```python
from build123d import *

# Parameters (mm, degrees)
SKETCH_1_W           = 50
SKETCH_1_H           = 50
EXTRUDE_1_DEPTH      = 50
SKETCH_6_R           = 12
SKETCH_6_R_2         = 11
EXTRUDE_3_DEPTH      = 9
CUT_EXTRUDE_5_REACH  = 83.277
CUT_EXTRUDE_6_REACH  = 83.277
SKETCH_20_W          = 48
SKETCH_20_H          = 48
CUT_EXTRUDE_7_DEPTH  = 30
CUT_EXTRUDE_START    = -29
SKETCH_21_R          = 11
CUT_EXTRUDE_9_DEPTH  = 29
SKETCH_28_W          = 48
SKETCH_28_H          = 48
CUT_EXTRUDE_11_DEPTH = 18
CUT_EXTRUDE_11_DRAFT = -33


with BuildPart() as part:
    # Эскиз1 → Бобышка-Вытянуть1 (new body)
    with BuildSketch(Plane.XY):
        Rectangle(SKETCH_1_W, SKETCH_1_H)
    extrude(amount=EXTRUDE_1_DEPTH)

    # Эскиз6 → Бобышка-Вытянуть3 (add)
    with BuildSketch(Plane.XY.offset(50)):
        Circle(SKETCH_6_R)
        Circle(SKETCH_6_R_2, mode=Mode.SUBTRACT)
    extrude(amount=EXTRUDE_3_DEPTH)

    # Вырез-Вытянуть5: up to this face of the body (flat: up to its plane)
    cut_extrude_5_end = Plane(part.part.faces().sort_by_distance((0, 25, 25))[0])
    # Эскиз19 → Вырез-Вытянуть5 (cut, up to the picked face)
    with BuildSketch(Plane.XZ.offset(25), mode=Mode.PRIVATE) as cut_extrude_5_sk1:
        Polygon((-12, 50), (-25, 50), (-25, 30), align=None)
    cut_extrude_5_tool1 = split(extrude(cut_extrude_5_sk1.sketch, amount=-CUT_EXTRUDE_5_REACH, mode=Mode.PRIVATE), bisect_by=cut_extrude_5_end, keep=Keep.BOTH, mode=Mode.PRIVATE)
    # Эскиз19 → Вырез-Вытянуть5 (cut, up to the picked face)
    with BuildSketch(Plane.XZ.offset(25), mode=Mode.PRIVATE) as cut_extrude_5_sk2:
        Polygon((12, 50), (25, 50), (25, 30), align=None)
    cut_extrude_5_tool2 = split(extrude(cut_extrude_5_sk2.sketch, amount=-CUT_EXTRUDE_5_REACH, mode=Mode.PRIVATE), bisect_by=cut_extrude_5_end, keep=Keep.BOTH, mode=Mode.PRIVATE)
    add(cut_extrude_5_tool1.solids().sort_by(Axis((-20.666667, -25, 43.333333), (0, 1, 0)))[0], mode=Mode.SUBTRACT)
    add(cut_extrude_5_tool2.solids().sort_by(Axis((20.666667, -25, 43.333333), (0, 1, 0)))[0], mode=Mode.SUBTRACT)

    # Вырез-Вытянуть6: up to this face of the body (flat: up to its plane)
    cut_extrude_6_end = Plane(part.part.faces().sort_by_distance((-25, 0, 15))[0])
    # Эскиз18 → Вырез-Вытянуть6 (cut, up to the picked face)
    with BuildSketch(Plane(origin=(25, 0, 0), x_dir=(0, 0, -1), z_dir=(1, 0, 0)), mode=Mode.PRIVATE) as cut_extrude_6_sk1:
        Polygon((-50, 12), (-50, 25), (-30, 25), align=None)
    cut_extrude_6_tool1 = split(extrude(cut_extrude_6_sk1.sketch, amount=-CUT_EXTRUDE_6_REACH, mode=Mode.PRIVATE), bisect_by=cut_extrude_6_end, keep=Keep.BOTH, mode=Mode.PRIVATE)
    # Эскиз18 → Вырез-Вытянуть6 (cut, up to the picked face)
    with BuildSketch(Plane(origin=(25, 0, 0), x_dir=(0, 0, -1), z_dir=(1, 0, 0)), mode=Mode.PRIVATE) as cut_extrude_6_sk2:
        Polygon((-50, -12), (-50, -25), (-30, -25), align=None)
    cut_extrude_6_tool2 = split(extrude(cut_extrude_6_sk2.sketch, amount=-CUT_EXTRUDE_6_REACH, mode=Mode.PRIVATE), bisect_by=cut_extrude_6_end, keep=Keep.BOTH, mode=Mode.PRIVATE)
    add(cut_extrude_6_tool1.solids().sort_by(Axis((25, 20.666667, 43.333333), (-1, 0, 0)))[0], mode=Mode.SUBTRACT)
    add(cut_extrude_6_tool2.solids().sort_by(Axis((25, -20.666667, 43.333333), (-1, 0, 0)))[0], mode=Mode.SUBTRACT)

    # Эскиз20 → Вырез-Вытянуть7 (cut)
    with BuildSketch(Plane(origin=(0, 0, 0), x_dir=(-1, 0, 0), z_dir=(0, 0, -1))):
        Rectangle(SKETCH_20_W, SKETCH_20_H)
    extrude(amount=-CUT_EXTRUDE_7_DEPTH, mode=Mode.SUBTRACT)

    # Эскиз21 → Вырез-Вытянуть9 (cut)
    with BuildSketch(Plane.XY.offset(59).offset(CUT_EXTRUDE_START)):
        Circle(SKETCH_21_R)
    extrude(amount=CUT_EXTRUDE_9_DEPTH, mode=Mode.SUBTRACT)


with BuildPart() as cut_extrude_11_tool:
    # Эскиз28 → Вырез-Вытянуть11 (with draft: the straight prism first)
    with BuildSketch(Plane(origin=(0, 0, 30), x_dir=(-1, 0, 0), z_dir=(0, 0, -1))):
        Rectangle(SKETCH_28_W, SKETCH_28_H)
    extrude(amount=-CUT_EXTRUDE_11_DEPTH)
    # Вырез-Вытянуть11: the draft: its side faces are tilted about the plane it starts from
    cut_extrude_11_sides = [cut_extrude_11_tool.faces().sort_by_distance(p)[0] for p in [
        (24, 0, 39),
        (0, -24, 39),
        (-24, 0, 39),
        (0, 24, 39),
    ]]
    draft(cut_extrude_11_sides, Plane(origin=(0, 0, 30), x_dir=(-1, 0, 0), z_dir=(0, 0, -1)), CUT_EXTRUDE_11_DRAFT)


with BuildPart() as part_1:
    add(part.part)

    # Вырез-Вытянуть11: cut by cut_extrude_11_tool
    add(cut_extrude_11_tool.part, mode=Mode.SUBTRACT)


solid = part_1.part
```
Geometry: final body of the model. Coordinates: model frame, mm. A direction names the side the tool comes from. Round coordinates to 2 decimals unless told otherwise and drop trailing zeros. Write each loop counter-clockwise with the first axis right and the second up, starting at its lowest first coordinate (ties: lowest second). Pieces come first, ordered by that corner, then holes. Notation, with made-up numbers: M 63,38 L 74,38 A33 ccw 74,66 Z; hole C 19.25,65 d11. An arc over 180 degrees is marked long. Answer in a Markdown table with one row per item. Add a question column.
(1) Reachability of faces 1 (the face through (-11.99, 0.53, 54.44)), 2 (the face through (24, 0, 15)), 3 (the face through (9, 10, 50)) from +Z, -Z, +X, -X, +Y, -Y: full face, straight path, thin tool, end or side. Return the list, or none.
(2) Cut plane D-D, the plane x = 14.5. Return the cut outline in (y, z).
(3) Cut plane C-C, the plane y = -19.5. Return the cut outline in (x, z).
(4) Cut plane A-A, the plane x = -7. Return the cut outline in (y, z).
(5) Draft query along X for faces 4 (the face through (20.035, -0.35, 37.638)), 5 (the face through (-25, 0, 15)), 6 (the face through (0.35, -20.035, 37.638)), 7 (the face through (-19.54, -0.34, 36.87)). Return one class per face: pulls with the +X half, pulls with the -X half, needs draft (parallel to the pull), parting line crosses it, or undercut.
(6) Cut plane B-B, the plane z = 21. Return the cut outline in (x, y).
(7) Contact query for flat-ended pins moving along their axis: pin 1 (19.5 mm diameter, centred on x = -4.5, y = 1.5, fed in from -Z); pin 2 (5 mm diameter, centred on y = -13.5, z = 47, fed in from -X) (3 decimals); pin 3 (8 mm diameter, centred on y = 8, z = 41.5, fed in from +X) (3 decimals); pin 4 (20 mm diameter, centred on x = 0, y = 0, fed in from -Z). Output: stop coordinate, or through.
(8) Ray query, L1, parallel to Y at x = -21, z = 28; L2, parallel to Y at x = 0, z = 55.75. Return the intervals inside material, ascending.
Established:
| question | item | result |
|---|---|---|
| 1 | face 1 | +Z |
| 1 | face 2 | -Z |
| 1 | face 3 | +Z, +X, +Y |
| 2 | outline | M -25,0 L -24,0 L -24,30 L -14.5,44.63 L 14.5,44.63 L 24,30 L 24,0 L 25,0 L 25,30 L 14.5,46.15 L -14.5,46.15 L -25,30 Z |
| 3 | outline | M -25,0 L -24,0 L -24,30 L -19.5,36.93 L 19.5,36.93 L 24,30 L 24,0 L 25,0 L 25,30 L 19.5,38.46 L -19.5,38.46 L -25,30 Z |
| 4 | outline | M -25,0 L -24,0 L -24,30 L -12.31,48 L -8.49,48 L -8.49,59 L -9.75,59 L -9.75,50 L -12,50 L -25,30 Z; M 8.49,48 L 12.31,48 L 24,30 L 24,0 L 25,0 L 25,30 L 12,50 L 9.75,50 L 9.75,59 L 8.49,59 Z |
| 5 | face 4 | pulls with the +X half |
| 5 | face 5 | pulls with the -X half |
| 5 | face 6 | needs draft |
| 5 | face 7 | undercut |
| 6 | outline | M -25,-25 L 25,-25 L 25,25 L -25,25 Z; hole M -24,-24 L 24,-24 L 24,24 L -24,24 Z |
| 7 | pin 1 | z = 45.01 |
| 7 | pin 2 | x = -15.575 |
| 7 | pin 3 | x = 20.125 |
| 7 | pin 4 | through |
| 8 | L1 | -25 to -24, 24 to 25 |
| 8 | L2 | -12 to -11, 11 to 12 |
